from build123d import *

# Parameters (mm, degrees)
SKETCH1_W           = 65
SKETCH1_H           = 56
BOSS_EXTRUDE1_DEPTH = 23
SKETCH2_W           = 57
SKETCH2_H           = 48
CUT_EXTRUDE1_DEPTH  = 20
SKETCH5_W           = 9
SKETCH5_H           = 13
CUT_EXTRUDE2_DEPTH  = 75.417739821


with BuildPart() as part:
    # Sketch1 → Boss-Extrude1 (new body)
    with BuildSketch(Plane.XY):
        Rectangle(SKETCH1_W, SKETCH1_H)
    extrude(amount=BOSS_EXTRUDE1_DEPTH)

    # Sketch2 → Cut-Extrude1 (cut)
    with BuildSketch(Plane.XY.offset(23)):
        Rectangle(SKETCH2_W, SKETCH2_H)
    extrude(amount=-CUT_EXTRUDE1_DEPTH, mode=Mode.SUBTRACT)

    # Sketch5 → Cut-Extrude2 (cut, through all)
    with BuildSketch(Plane.ZY.offset(32.5)):
        with Locations((10.5, -13.5)):
            Rectangle(SKETCH5_W, SKETCH5_H)
    extrude(amount=-CUT_EXTRUDE2_DEPTH, mode=Mode.SUBTRACT)


solid = part.part
Model file for the job. Use its own axes, mm. A direction names the side the tool comes from. Give positions to 0.01 mm unless a question says otherwise; leave off trailing zeros. Write each loop counter-clockwise with the first axis right and the second up, starting at its lowest first coordinate (ties: lowest second). Pieces come first, ordered by that corner, then holes. Notation, with made-up numbers: (17, 2) -> (30, 2) arc R35 ccw to (30, 38) -> close; hole circle Ø2 at (-25.75, -24). An arc over 180 degrees is marked (long way). Write item = value, one per line.
(1) Mould opens along X. For faces 4 (the face through (-28.5, 0, 13)), 5 (the face through (0, 0, 3)), 6 (the face through (-31, -14, 15)), 7 (the face through (-32.5, 0, 11)) say: released by +X, released by -X, zero draft, split by the parting line, or undercut.
Determined:
face_4 = undercut
face_5 = undercut
face_6 = zero draft
face_7 = released by -X
(2) Flat gauge pins, fed straight in: P1, Ø2, axis at x = 30.5, y = -11.5, coming from the -Z side; P2, Ø1, axis at x = 9.5, y = -3, coming from the +Z side. Where does each tip first touch, or does it go through?
Determined:
P1 = 0
P2 = 3
(3) Slice it at A-A, the plane z = 14. Give the cut face in (x, y).
Determined:
outline = (-32.5, -28) -> (32.5, -28) -> (32.5, -20) -> (28.5, -20) -> (28.5, -24) -> (-28.5, -24) -> (-28.5, -20) -> (-32.5, -20) -> close; (-32.5, -7) -> (-28.5, -7) -> (-28.5, 24) -> (28.5, 24) -> (28.5, -7) -> (32.5, -7) -> (32.5, 28) -> (-32.5, 28) -> close
(4) Slice it at B-B, the plane x = 17. Give the cut face in (y, z), then the cut area to 3 significant figures.
Determined:
outline = (-28, 0) -> (28, 0) -> (28, 23) -> (24, 23) -> (24, 3) -> (-24, 3) -> (-24, 23) -> (-28, 23) -> close
area = 328 mm2
(5) Slice it at C-C, the plane y = 1.5. Give the cut face in (x, z), then the cut area to 3 significant figures.
Determined:
outline = (-32.5, 0) -> (32.5, 0) -> (32.5, 23) -> (28.5, 23) -> (28.5, 3) -> (-28.5, 3) -> (-28.5, 23) -> (-32.5, 23) -> close
area = 355 mm2
(6) Probe line 1 along X through (y, z) = (-12.5, 18.5); line 2 along Y through (x, z) = (26.5, 11); line 3 along Z through (x, y) = (-12.5, 14.5). List the from-to ranges inside material, lowest first.
Determined:
line_1 = -32.5 to -28.5, 28.5 to 32.5
line_2 = -28 to -24, 24 to 28
line_3 = 0 to 3
(7) Tool access for faces 1 (the face through (30, -14, 15)), 2 (the face through (28.5, 0, 13)), 3 (the face through (32.5, 0, 11)): list every direction of +Z, -Z, +X, -X, +Y, -Y with a clear straight run to the whole face (end or side of a thin tool).
Determined:
face_1 = +X, -X
face_2 = +Z
face_3 = +Z, -Z, +X, +Y, -Y
